Check sheet for the modelled part. Datum: model origin and axes. Units: mm. Round coordinates to 2 decimals unless told otherwise and drop trailing zeros. Write each loop counter-clockwise with the first axis right and the second up, starting at its lowest first coordinate (ties: lowest second). Pieces come first, ordered by that corner, then holes.
Item 1: Cross-section at A-A on x = -2.6. Enter the section's corners in (y, z).
Item 2: Cross-section at D-D on x = 0.6. Enter the section's corners in (y, z).
Item 3: Cross-section at B-B on y = 0. Enter the section's corners in (x, z), plus the area to 3 significant figures.
Item 4: Cross-section at C-C on z = -3. Enter the section's corners in (x, y), plus the area to 3 significant figures.
Item 5: Material ranges on line 1 (Z direction, x = -0.5, y = -0.1); line 2 (Z direction, x = -2.2, y = 0); line 3 (Z direction, x = -2.05, y = 0.15), recorded low to high.
from build123d import *

# Parameters (mm, degrees)
SKETCH1_R           = 1
BOSS_EXTRUDE1_DEPTH = 1.5
DOME1_FACE_RADIUS   = 1
DOME1_HEIGHT        = 1
DOME2_FACE_RADIUS   = 1
DOME2_HEIGHT        = 1
SKETCH4_R           = 0.25


with BuildPart() as part:
    # Sketch1 → Boss-Extrude1 (new, symmetric)
    with BuildSketch(Plane.XY):
        Circle(SKETCH1_R)
    extrude(amount=BOSS_EXTRUDE1_DEPTH, both=True)

    # Dome1: a dome of height H over a round flat face of radius A is a cap of a sphere of radius (A * A + H * H) / (2 * H)
    dome1_r = (DOME1_FACE_RADIUS * DOME1_FACE_RADIUS + DOME1_HEIGHT * DOME1_HEIGHT) / (2 * DOME1_HEIGHT)
    dome1_base = Plane((0, 0, 1.5), z_dir=(0, 0, 1))
    with Locations(dome1_base.offset(DOME1_HEIGHT - dome1_r)):
        dome1_ball = Sphere(dome1_r, mode=Mode.PRIVATE)
    add(split(dome1_ball, bisect_by=dome1_base, keep=Keep.TOP, mode=Mode.PRIVATE))

    # Dome2: a dome of height H over a round flat face of radius A is a cap of a sphere of radius (A * A + H * H) / (2 * H)
    dome2_r = (DOME2_FACE_RADIUS * DOME2_FACE_RADIUS + DOME2_HEIGHT * DOME2_HEIGHT) / (2 * DOME2_HEIGHT)
    dome2_base = Plane((0, 0, -1.5), z_dir=(0, 0, -1))
    with Locations(dome2_base.offset(DOME2_HEIGHT - dome2_r)):
        dome2_ball = Sphere(dome2_r, mode=Mode.PRIVATE)
    add(split(dome2_ball, bisect_by=dome2_base, keep=Keep.TOP, mode=Mode.PRIVATE))

    # Sweep1: sweep along a path in Sketch3
    with BuildLine(Plane(origin=(0, 0, 0), x_dir=(1, 0, 0), z_dir=(0, 1, 0))) as sweep1_path:
        Line((-3, -5.08), (-1.2, -5.08))
        ThreePointArc((-1.2, -5.08), (-0.351471863, -4.728528137), (0, -3.88))
        Line((0, -3.88), (0, 3.88))
        ThreePointArc((0, 3.88), (-0.351471863, 4.728528137), (-1.2, 5.08))
        Line((-1.2, 5.08), (-3, 5.08))
    # Sketch4 → Sweep1 (sweep)
    with BuildSketch(Plane.XY):
        Circle(SKETCH4_R)
    sweep(path=sweep1_path.line)


solid = part.part
Response values:
1. outline: circle Ø0.5 at (0, -5.08); circle Ø0.5 at (0, 5.08)
2. outline: (-0.8, -1.5) arc R0.8 ccw to (0.8, -1.5) - (0.8, 1.5) arc R0.8 ccw to (-0.8, 1.5) - close
3. outline: (-3, -5.33) - (-1.2, -5.33) arc R1.45 ccw to (0.25, -3.88) - (0.25, -2.47) arc R1 ccw to (1, -1.5) - (1, 1.5) arc R1 ccw to (0.25, 2.47) - (0.25, 3.88) arc R1.45 ccw to (-1.2, 5.33) - (-3, 5.33) - (-3, 4.83) - (-1.2, 4.83) arc R0.95 cw to (-0.25, 3.88) - (-0.25, 2.47) arc R1 ccw to (-1, 1.5) - (-1, -1.5) arc R1 ccw to (-0.25, -2.47) - (-0.25, -3.88) arc R0.95 cw to (-1.2, -4.83) - (-3, -4.83) - close
3. area: 14.2 mm2
4. outline: circle Ø0.5 at (0, 0)
4. area: 0.196 mm2
5. line 1: z = -5.13 to -4.55, -2.36 to 2.36, 4.55 to 5.13
5. line 2: z = -5.33 to -4.83, 4.83 to 5.33
5. line 3: z = -5.28 to -4.88, 4.88 to 5.28
